CAD build for the part. Positions are in the model's coordinates, mm. Face numbers are marked on the shaded views. A direction names the side the tool comes from. Coordinates: 2 decimals unless noted, no trailing zeros. Order: outer loops, then holes, each group sorted by start corner. A loop starts at its lowest first (then second) coordinate and runs counter-clockwise, first axis right, second up. Notation, with made-up numbers: M 21,0 L 58,0 A21 ccw 58,11 Z; hole C 84.5,-12 d3. An arc over 180 degrees is marked long. One line per item, written item: value.
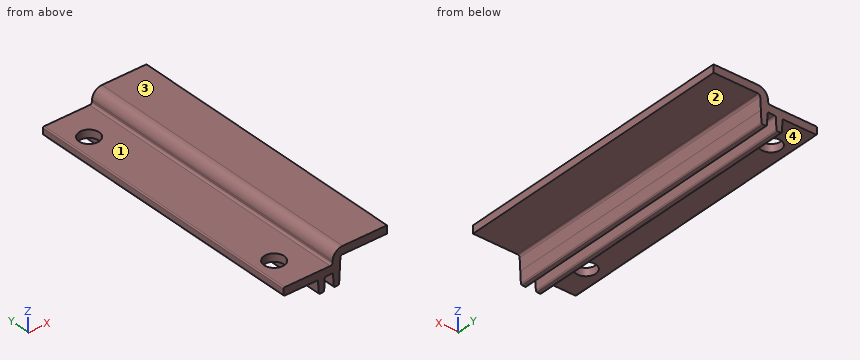
from build123d import *

# Parameters (mm, degrees)
F1_DEPTH = 130
F3_D     = 9
F4_D     = 9


with BuildPart() as f1:
    # F0 (on Front) → F1 (new body)
    with BuildSketch(Plane.XZ):
        with BuildLine():
            Line((25, -6.026168), (25.264782, -0.973832))
            Line((25.264782, -0.973832), (25.554396, 4.552336))
            ThreePointArc((25.554396, 4.552336), (25.864671, 5.225374), (26.553025, 5.5))
            Line((26.553025, 5.5), (46.553025, 5.5))
            Line((46.553025, 5.5), (46.553025, 9))
            Line((46.553025, 9), (26.553025, 9))
            ThreePointArc((26.553025, 9), (23.45543, 7.764185), (22.059193, 4.735512))
            Line((22.059193, 4.735512), (22.017903, 3.947664))
            ThreePointArc((22.017903, 3.947664), (21.707628, 3.274626), (21.019274, 3))
            Line((21.019274, 3), (0.5, 3))
            ThreePointArc((0.5, 3), (0.146447, 2.853553), (0, 2.5))
            Line((0, 2.5), (0, 0))
            ThreePointArc((0, 0), (0.146447, -0.353553), (0.5, -0.5))
            Line((0.5, -0.5), (15.025467, -0.5))
            ThreePointArc((15.025467, -0.5), (15.369644, -0.637313), (15.524782, -0.973832))
            Line((15.524782, -0.973832), (15.789563, -6.026168))
            ThreePointArc((15.789563, -6.026168), (15.944701, -6.362687), (16.288878, -6.5))
            Line((16.288878, -6.5), (17.760685, -6.5))
            ThreePointArc((17.760685, -6.5), (18.104863, -6.362687), (18.26, -6.026168))
            Line((18.26, -6.026168), (18.524782, -0.973832))
            ThreePointArc((18.524782, -0.973832), (18.679919, -0.637313), (19.024096, -0.5))
            Line((19.024096, -0.5), (21.765467, -0.5))
            ThreePointArc((21.765467, -0.5), (22.109644, -0.637313), (22.264782, -0.973832))
            Line((22.264782, -0.973832), (22.529563, -6.026168))
            ThreePointArc((22.529563, -6.026168), (22.684701, -6.362687), (23.028878, -6.5))
            Line((23.028878, -6.5), (24.500685, -6.5))
            ThreePointArc((24.500685, -6.5), (24.844863, -6.362687), (25, -6.026168))
        make_face()
    extrude(amount=F1_DEPTH)

    # F3 (through all)
    with Locations(Plane(origin=(0, 0, -0.5), x_dir=(1, 0, 0), z_dir=(0, 0, -1))):
        with Locations((8.25, 115)):
            Hole(F3_D / 2)

    # F4 (through all)
    with Locations(Plane(origin=(0, 0, -0.5), x_dir=(1, 0, 0), z_dir=(0, 0, -1))):
        with Locations((8.25, 15)):
            Hole(F4_D / 2)


solid = f1.part
Q1. Pin check, flat tips, straight feed: pin 1 Ø22 at (x, y) = (32.5, -64) entering from -Z; pin 2 Ø1.4 at (x, y) = (21, -89.5) entering from -Z; pin 3 Ø4 at (y, z) = (-25, 0) entering from +X; pin 4 Ø14.5 at (x, y) = (8.25, -15) entering from +Z. Stop position of each tip, or through.
Recorded:
pin 1: stops at z = -6.5
pin 2: stops at z = -0.5
pin 3: stops at x = 25.42
pin 4: stops at z = 3
Q2. Drill centre lines: line 1 along Y through (x, z) = (8.25, 2.15); line 2 along Y through (x, z) = (9, 1.75); line 3 along Z through (x, y) = (13, -116). Where is each one in solid material? Low to high.
Recorded:
line 1: y = -130 to -119.5, -110.5 to -19.5, -10.5 to 0
line 2: y = -130 to -119.44, -110.56 to -19.44, -10.56 to 0
line 3: z = -0.5 to 3
Q3. Slice it at C-C (z = -4). List the corners of the cut face in (x, y).
Recorded:
outline: M 15.68,-130 L 18.37,-130 L 18.37,0 L 15.68,0 Z; M 22.42,-130 L 25.11,-130 L 25.11,0 L 22.42,0 Z
Q4. Slice it at D-D (x = 40). List the corners of the cut face in (y, z).
Recorded:
outline: M -130,5.5 L 0,5.5 L 0,9 L -130,9 Z
Q5. Slice it at B-B (x = 8.25). List the corners of the cut face in (y, z), plus the area to 3 significant figures.
Recorded:
outline: M -130,-0.5 L -119.5,-0.5 L -119.5,3 L -130,3 Z; M -110.5,-0.5 L -19.5,-0.5 L -19.5,3 L -110.5,3 Z; M -10.5,-0.5 L 0,-0.5 L 0,3 L -10.5,3 Z
area: 392 mm^2
Q6. Which spindle directions (+Z, -Z, +X, -X, +Y, -Y) get a long thin tool onto all of the face, cutting with end or side? Do the marked faces 1, 2, 3 and 4. Say none if no direction does.
Recorded:
face 1: +Z, -X, +Y, -Y
face 2: -Z, +X, +Y, -Y
face 3: +Z, +X, -X, +Y, -Y
face 4: -Z, -X, +Y, -Y
